from build123d import *

# Parameters (mm, degrees)
F1_W      = 8
F1_H      = 16
F1_W_2    = 5
F1_H_2    = 13
F2_DEPTH  = 8
F3_W      = 8
F3_H      = 16
F3_W_2    = 5
F3_H_2    = 13
F4_DEPTH  = 1.5
F5_R      = 2.5
F5_R_2    = 1.75
F6_DEPTH  = 1.8
F8_DEPTH  = 7.9
F10_DEPTH = 25
F11_DEPTH = 0.5
F12_R     = 2.5
F12_R_2   = 2.25
F13_DEPTH = 0.5
F15_DEPTH = 4.2


with BuildPart() as f2:
    # F1 (on face) → F2 (new body)
    with BuildSketch(Plane.XY):
        with Locations((-31.9046421945, 0.9305412807)):
            Rectangle(F1_W, F1_H)
        with Locations((-31.9046421945, 0.9305412807)):
            Rectangle(F1_W_2, F1_H_2, mode=Mode.SUBTRACT)
    extrude(amount=F2_DEPTH)

    # F3 (on face) → F4 (join)
    with BuildSketch(Plane.XY.offset(8)):
        with Locations((-31.9046421945, 0.9305412807)):
            Rectangle(F3_W, F3_H)
        with Locations((-31.9046421945, 0.9305412807)):
            Rectangle(F3_W_2, F3_H_2, mode=Mode.SUBTRACT)
        with Locations((-31.9046421945, 0.9305412807)):
            Rectangle(F3_W_2, F3_H_2)
    extrude(amount=F4_DEPTH)

    # F5 (on face) → F6 (join)
    with BuildSketch(Plane.XY.offset(9.5)):
        with Locations((-31.9046421945, -3.0694587193)):
            Circle(F5_R)
        with Locations((-31.9046421945, -3.0694587193)):
            Circle(F5_R_2, mode=Mode.SUBTRACT)
        with Locations((-31.9046421945, 4.9305412807)):
            Circle(F5_R)
        with Locations((-31.9046421945, 4.9305412807)):
            Circle(F5_R_2, mode=Mode.SUBTRACT)
    extrude(amount=F6_DEPTH)

    # F7 (on face) → F8 (join)
    with BuildSketch(Plane.YZ.offset(-27.9046421945)):
        with BuildLine():
            ThreePointArc((0.9305412807, 9.5), (-1.1907790629, 4.3786796564), (3.9305412807, 6.5))
            ThreePointArc((3.9305412807, 6.5), (3.0518616242, 8.6213203436), (0.9305412807, 9.5))
        make_face()
    extrude(amount=-F8_DEPTH)

    # F9 (on face) → F10 (cut)
    with BuildSketch(Plane.YZ.offset(-27.9046421945)):
        with BuildLine():
            ThreePointArc((3.1805412807, 6.5), (2.5215315383, 8.0909902577), (0.9305412807, 8.75))
            ThreePointArc((0.9305412807, 8.75), (-0.660448977, 4.9090097423), (3.1805412807, 6.5))
        make_face()
    extrude(amount=-F10_DEPTH, mode=Mode.SUBTRACT)

    # F9 (on face) → F11 (cut)
    with BuildSketch(Plane.YZ.offset(-27.9046421945)):
        with BuildLine():
            ThreePointArc((0.9305412807, 9), (-0.8372256723, 4.732233047), (3.4305412807, 6.5))
            ThreePointArc((3.4305412807, 6.5), (2.6983082336, 8.267766953), (0.9305412807, 9))
        make_face()
        with BuildLine():
            ThreePointArc((3.1805412807, 6.5), (-0.660448977, 4.9090097423), (0.9305412807, 8.75))
            ThreePointArc((0.9305412807, 8.75), (2.5215315383, 8.0909902577), (3.1805412807, 6.5))
        make_face(mode=Mode.SUBTRACT)
    extrude(amount=-F11_DEPTH, mode=Mode.SUBTRACT)

    # F12 (on face) → F13 (cut)
    with BuildSketch(Plane(origin=(-35.9046421945, 0, 0), x_dir=(0, -1, 0), z_dir=(-1, 0, 0))):
        with Locations((-0.9305412807, 6.5)):
            Circle(F12_R)
        with Locations((-0.9305412807, 6.5)):
            Circle(F12_R_2, mode=Mode.SUBTRACT)
    extrude(amount=-F13_DEPTH, mode=Mode.SUBTRACT)

    # F14 (on Top) → F15 (join)
    with BuildSketch(Plane.XY):
        with BuildLine():
            ThreePointArc((-30.4045602381, 0.9304907289), (-31.9045602381, 2.4304907289), (-33.4045602381, 0.9304907289))
            ThreePointArc((-33.4045602381, 0.9304907289), (-31.9045602381, -0.5695092711), (-30.4045602381, 0.9304907289))
        make_face()
        with BuildLine():
            ThreePointArc((-31.1545602381, 0.9304907289), (-31.9045602381, 0.1804907289), (-32.6545602381, 0.9304907289))
            ThreePointArc((-32.6545602381, 0.9304907289), (-31.9045602381, 1.6804907289), (-31.1545602381, 0.9304907289))
        make_face(mode=Mode.SUBTRACT)
    extrude(amount=F15_DEPTH)


solid = f2.part
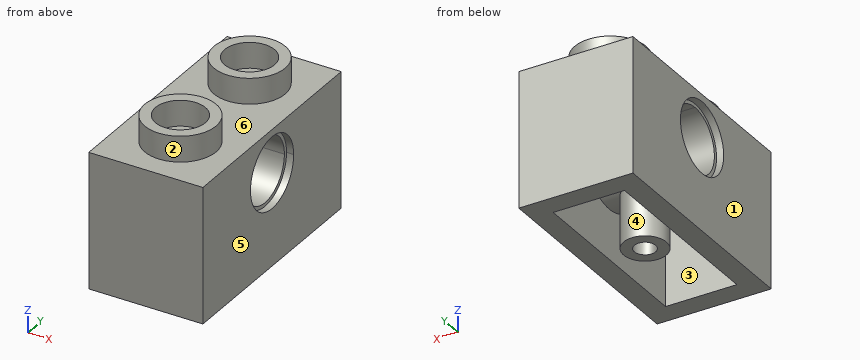
Work out the finished part from the listing and answer in its coordinate system (mm). Face numbers are marked on the shaded views. A direction names the side the tool comes from. Round coordinates to 2 decimals unless told otherwise and drop trailing zeros. Write each loop counter-clockwise with the first axis right and the second up, starting at its lowest first coordinate (ties: lowest second). Pieces come first, ordered by that corner, then holes. Notation, with made-up numbers: M 41,22.25 L 90,22.25 A20 ccw 90,34.25 Z; hole C 42.25,76 d3. An arc over 180 degrees is marked long. Use a Markdown table: item, result.
1) The part is cut by section A-A on z = 10. Give the vertices of the cut face in (x, y).
Taken from the geometry:
| item | result |
|---|---|
| outline | C -31.9,-3.07 d5; C -31.9,4.93 d5; hole C -31.9,-3.07 d3.5; hole C -31.9,4.93 d3.5 |
2) Flat-ended cylindrical pins translate along their axes: pin 1 (3 mm diameter, centred on x = -31.9, y = -3.07, fed in from -Z); pin 2 (2.5 mm diameter, centred on y = 2, z = 6, fed in from -X); pin 3 (2 mm diameter, centred on x = -31, y = -4.5, fed in from -Z). Find the tip coordinate at first contact, or state that the pin passes through.
Taken from the geometry:
| item | result |
|---|---|
| pin 1 | stops at z = 4.84 |
| pin 2 | stops at x = -35.4 |
| pin 3 | stops at z = 8 |
3) Which of the six approach directions +Z, -Z, +X, -X, +Y, -Y give full straight-line access (tool end or side, diameter ignored) to the marked faces 4, 5 and 6?
Taken from the geometry:
| item | result |
|---|---|
| face 4 | -Z |
| face 5 | +Z, -Z, +X, +Y, -Y |
| face 6 | +Z |
4) Consider line 1 (Y direction, x = -33, z = 6.5); line 2 (Y direction, x = -33.5, z = 2.75); line 3 (X direction, y = -3.5, z = 3). Determine where each line is inside the solid, lowest interval first. Write a range as [from, to].
Taken from the geometry:
| item | result |
|---|---|
| line 1 | y = [-7.07, -5.57], [-2.07, -1.32], [3.18, 3.93], [7.43, 8.93] |
| line 2 | y = [-7.07, -5.57], [7.43, 8.93] |
| line 3 | x = [-35.9, -34.4], [-29.4, -27.9] |
5) Determine the mould class of the marked faces 1, 2 and 3 for opening direction X: pulls with the +X half, pulls with the -X half, needs draft (parallel to the pull), parting line crosses it, or undercut.
Taken from the geometry:
| item | result |
|---|---|
| face 1 | pulls with the -X half |
| face 2 | parting line crosses it |
| face 3 | undercut |
6) The part is cut by section B-B on y = 6.25. Give the vertices of the cut face in (x, z).
Taken from the geometry:
| item | result |
|---|---|
| outline | M -35.9,0 L -34.4,0 L -34.4,8 L -29.4,8 L -29.4,0 L -27.9,0 L -27.9,9.5 L -29.78,9.5 L -29.78,11.3 L -30.76,11.3 L -30.76,9.5 L -33.05,9.5 L -33.05,11.3 L -34.03,11.3 L -34.03,9.5 L -35.9,9.5 Z |
